```python
from build123d import *

# Parameters (mm, degrees)
EXTRUDE_1_DEPTH              = 10
EXTRUDE_2_DEPTH              = 5
EXTRUDE_3_DEPTH              = 15
EXTRUDE_4_DEPTH              = 3
HOLE_WIZARD_M3_1_D           = 3.4
HOLE_WIZARD_M3_1_CSINK_D     = 6.3
HOLE_WIZARD_M3_1_CSINK_ANGLE = 90
HOLE_WIZARD_M3_1_2_D         = 3.15


with BuildPart() as part:
    # 草图1 → 凸台-拉伸1 (new body)
    with BuildSketch(Plane.XY):
        Polygon((0, 0), (20, 30), (30, 30), (30, 0), align=None)
    extrude(amount=EXTRUDE_1_DEPTH)

    # 草图2 → 凸台-拉伸2 (add)
    with BuildSketch(Plane.XZ):
        Polygon((0, 10), (30, 10), (30, 0), (15, -30), (0, -30), align=None)
    extrude(amount=EXTRUDE_2_DEPTH)

    # 草图3 → 凸台-拉伸3 (add)
    with BuildSketch(Plane.ZY):
        with BuildLine():
            Line((-30, -5), (-17.090434036, -42.444533735))
            ThreePointArc((-17.090434036, -42.444533735), (-10, -47.5), (-2.909565964, -42.444533735))
            Line((-2.909565964, -42.444533735), (10, -5))
            Line((10, -5), (-30, -5))
        make_face()
    extrude(amount=-EXTRUDE_3_DEPTH)

    # 草图4 → 凸台-拉伸4 (add)
    with BuildSketch(Plane(origin=(0, 0, 0), x_dir=(1, 0, 0), z_dir=(0, 1, 0))):
        Polygon((0, 11), (24.5, 11), (20.5, 19), (0, 19), align=None)
    extrude(amount=EXTRUDE_4_DEPTH)

    # Hole Wizard M3 _1 (through all)
    with Locations(Plane.XY.offset(10)):
        with Locations((25, 15)):
            CounterSinkHole(HOLE_WIZARD_M3_1_D / 2, HOLE_WIZARD_M3_1_CSINK_D / 2, counter_sink_angle=HOLE_WIZARD_M3_1_CSINK_ANGLE)

    # Hole Wizard M3 _1 2 (through all)
    with Locations(Plane.ZY):
        with Locations((-10, -40)):
            Hole(HOLE_WIZARD_M3_1_2_D / 2)


solid = part.part
```
For this review, take the finished solid that the model builds, in its own axes (mm). A direction names the side the tool comes from. Give positions to 0.01 mm unless a question says otherwise; leave off trailing zeros. Write each loop counter-clockwise with the first axis right and the second up, starting at its lowest first coordinate (ties: lowest second). Pieces come first, ordered by that corner, then holes. Notation, with made-up numbers: M 49,-5.5 L 104,-5.5 A31 cw 104,18.5 Z; hole C 49,-17.5 d5. An arc over 180 degrees is marked long. One line per item, written item: value.
1) Take a section at B-B, the plane y = 15. Write out the cut boundary in (x, z), then the cut area to 3 significant figures.
Results are:
outline: M 10,0 L 23.3,0 L 23.3,8.55 L 21.85,10 L 10,10 Z; M 26.7,0 L 30,0 L 30,10 L 28.15,10 L 26.7,8.55 Z
area: 164 mm²
2) For line 1 (X direction, y = 15, z = 5); line 2 (Z direction, x = 15, y = 2); line 3 (Y direction, x = 25, z = 4.5), list the stretches that pass through material, from the lowest coordinate up. Write a range as from..to.
Results are:
line 1: x = 10..23.3, 26.7..30
line 2: z = -19..-11, 0..10
line 3: y = -5..13.3, 16.7..30
3) Take a section at D-D, the plane x = 6.5. Write out the cut boundary in (y, z) (3 decimals).
Results are:
outline: M -42.445,-17.09 L -5,-30 L 0,-30 L 0,-19 L 3,-19 L 3,-11 L 0,-11 L 0,0 L 9.75,0 L 9.75,10 L -5,10 L -42.445,-2.91 A7.5 ccw Z; hole C -40,-10 d3.15
4) For faces 1 (the flat face through (8, 0, -24)), 2 (the flat face through (12, 1, -11)), 3 (the flat face through (7.395, -23.46, -23.636)), 4 (the cylindrical face through (7.605, -38.936, -8.839)), 5 (the flat face through (15, -21, -10)), list the 3-axis set-ups (+Z, -Z, +X, -X, +Y, -Y) from which the entire face can be reached by the end or side of a thin tool; tool diameter is ignored.
Results are:
face 1: -Z, +X, -X, +Y
face 2: +X, -X, +Y
face 3: -Z, +X, -X, -Y
face 4: +X, -X
face 5: +Z, -Z, +X, -Y
5) Take a section at A-A, the plane x = 3. Write out the cut boundary in (y, z) (3 decimals), then the cut area to 3 significant figures.
Results are:
outline: M -42.445,-17.09 L -5,-30 L 0,-30 L 0,-19 L 3,-19 L 3,-11 L 0,-11 L 0,0 L 4.5,0 L 4.5,10 L -5,10 L -42.445,-2.91 A7.5 ccw Z; hole C -40,-10 d3.15
area: 1,330 mm²
6) For P1, Ø5, axis at x = 16.5, y = -27, coming from the -Z side; P2, Ø12, axis at x = 7, y = 19.5, coming from the -Z side; P3, Ø1.5, axis at x = 10.5, y = 2, coming from the -Z side; P4, Ø3, axis at y = -40, z = -10, coming from the -X side, all flat-tipped, find the tip position at first contact; note any pin that passes through.
Results are:
P1: stops at z = -23.1
P2: stops at z = 0
P3: stops at z = -19
P4: passes through
7) The part is to be moulded in two halves that separate along X. For faces 6 (the flat face through (10, 1, -19)), 7 (the flat face through (0, -22, -10)), 8 (the cylindrical face through (23.43, 14.35, 4.22)), say which applies: +X half, -X half, draft (parallel to the pull), parting line (faces both ways), or undercut.
Results are:
face 6: draft
face 7: -X half
face 8: undercut
8) Take a section at C-C, the plane y = -4. Write out the cut boundary in (x, z).
Results are:
outline: M 0,-30 L 15,-30 L 30,0 L 30,10 L 0,10 Z
